Part print with two shaded views. Sizes in mm from the minimum x, y, z corner. A direction names the side the tool comes from. Round coordinates to 2 decimals unless told otherwise and drop trailing zeros. Order: outer loops, then holes, each group sorted by start corner. A loop starts at its lowest first (then second) coordinate and runs counter-clockwise, first axis right, second up. Notation, with made-up numbers: (26, 68) -> (58, 68) arc R15 cw to (58, 79) -> close; hole circle Ø8 at (75.5, -39). An arc over 180 degrees is marked (long way). Use a Markdown table: item, result. Add a question column.
Item 1: Slice it at D-D, the plane z = 20.5. Give the cut face in (x, y) (1 decimal), plus the area to 3 significant figures.
Item 2: Slice it at C-C, the plane y = 15.5. Give the cut face in (x, z).
Item 3: Slice it at A-A, the plane x = 34. Give the cut face in (y, z).
Item 4: 3-axis set-ups, long thin cutter, end or side, ignore diameter. For the marked faces 1 and 2: which of +Z, -Z, +X, -X, +Y, -Y reach the whole face in a straight line?
Item 5: Slice it at B-B, the plane z = 26.55. Give the cut face in (x, y), plus the area to 3 significant figures.
Item 6: Pin check, flat tips, straight feed: pin 1 (4.5 mm diameter, centred on y = 7.38, z = 11.05, fed in from -X); pin 2 (10 mm diameter, centred on y = 32, z = 19.5, fed in from +X); pin 3 (1.9 mm diameter, centred on x = 27.6, z = 3.2, fed in from +Y); pin 4 (3.5 mm diameter, centred on x = 14.8, z = 34.4, fed in from +Y). Stop position of each tip, or through.
Item 7: Probe L1, parallel to Y at x = 25.5, z = 26.5. List the from-to ranges inside material, lowest first.
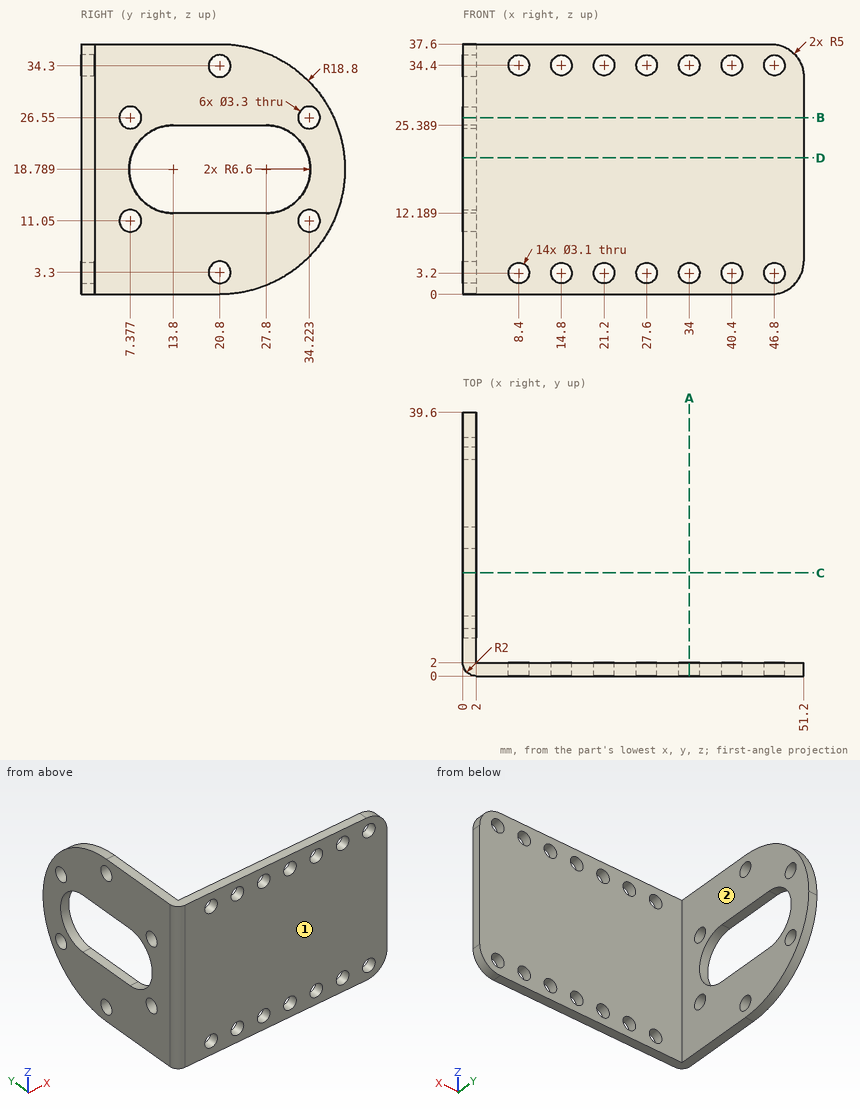
Check sheet entries:
| question | item | result |
|---|---|---|
| 1 | outline | (0, 2) arc R2 ccw to (2, 0) -> (51.2, 0) -> (51.2, 2) -> (2, 2) -> (2, 7.4) -> (0, 7.4) -> close; (0, 34.2) -> (2, 34.2) -> (2, 39.5) -> (0, 39.5) -> close |
| 1 | area | 123 mm2 |
| 2 | outline | (0, 0) -> (2, 0) -> (2, 12.19) -> (0, 12.19) -> close; (0, 25.39) -> (2, 25.39) -> (2, 37.6) -> (0, 37.6) -> close |
| 3 | outline | (0, 0) -> (2, 0) -> (2, 1.65) -> (0, 1.65) -> close; (0, 4.75) -> (2, 4.75) -> (2, 32.85) -> (0, 32.85) -> close; (0, 35.95) -> (2, 35.95) -> (2, 37.6) -> (0, 37.6) -> close |
| 4 | face 1 | +Z, -Z, +X, -X, -Y |
| 4 | face 2 | +Z, -Z, +X, +Y |
| 5 | outline | (0, 2) arc R2 ccw to (2, 0) -> (51.2, 0) -> (51.2, 2) -> (2, 2) -> (2, 5.73) -> (0, 5.73) -> close; (0, 9.03) -> (2, 9.03) -> (2, 32.57) -> (0, 32.57) -> close; (0, 35.87) -> (2, 35.87) -> (2, 37.93) -> (0, 37.93) -> close |
| 5 | area | 160 mm2 |
| 6 | pin 1 | x = 0 |
| 6 | pin 2 | x = 2 |
| 6 | pin 3 | through |
| 6 | pin 4 | y = 2 |
| 7 | L1 | 0 to 2 |
